```python
from build123d import *

# Parameters (mm, degrees)
BOSS_EXTRUDE1_DEPTH      = 47.064502155
BOSS_EXTRUDE1_DEPTH_BACK = 1
SKETCH1_W                = 107.713145043
SKETCH1_H                = 42.376311336
SKETCH2_R                = 13.469541987
SKETCH2_R_2              = 9.325857952
BOSS_EXTRUDE2_DEPTH      = 25.604576726
SKETCH3_OUTSIDE_W        = 137.154
SKETCH3_OUTSIDE_H        = 71.816
CUT_EXTRUDE2_DEPTH       = 12.802288363
SKETCH5_W                = 30.426797769
SKETCH5_H                = 5.633317916
CUT_EXTRUDE3_DEPTH       = 19.604576726


with BuildPart() as part:
    # Sketch1 → Boss-Extrude1 (new, two sides: drawn at the far end of the back side and taken through both)
    with BuildSketch(Plane(origin=(-41.279886751, 0, 0), x_dir=(1, 0, 0), z_dir=(0, 0, 1)).offset(-BOSS_EXTRUDE1_DEPTH_BACK)):
        with Locations((16.738942234, -3.835786802)):
            Rectangle(SKETCH1_W, SKETCH1_H)
    extrude(amount=BOSS_EXTRUDE1_DEPTH + BOSS_EXTRUDE1_DEPTH_BACK)

    # Sketch2 → Boss-Extrude2 (add)
    with BuildSketch(Plane(origin=(-44.843209588, 3.141572349, 47.064502155), x_dir=(1, 0, 0), z_dir=(0, 0, 1))):
        with Locations((1.586562206, -2.539630295)):
            Circle(SKETCH2_R)
        with Locations((1.586562206, -2.539630295)):
            Circle(SKETCH2_R_2, mode=Mode.SUBTRACT)
    extrude(amount=BOSS_EXTRUDE2_DEPTH)

    # Sketch3 outside → Cut-Extrude2 (cut, symmetric)
    with BuildSketch(Plane.XY.offset(72.669078881)):
        with Locations((-24.541, -3.836)):
            Rectangle(SKETCH3_OUTSIDE_W, SKETCH3_OUTSIDE_H)
        Polygon((-18.492947879, -30.338784684), (-15.338367542, -1.062929581), (-42.269291948, -12.968910423), align=None, mode=Mode.SUBTRACT)
    extrude(amount=CUT_EXTRUDE2_DEPTH, both=True, mode=Mode.SUBTRACT)

    # Sketch5 → Cut-Extrude3 (cut)
    with BuildSketch(Plane.XY.offset(47.064502155)):
        with Locations((7.480827718, 6.71069858)):
            Rectangle(SKETCH5_W, SKETCH5_H)
    extrude(amount=-CUT_EXTRUDE3_DEPTH, mode=Mode.SUBTRACT)


solid = part.part
```
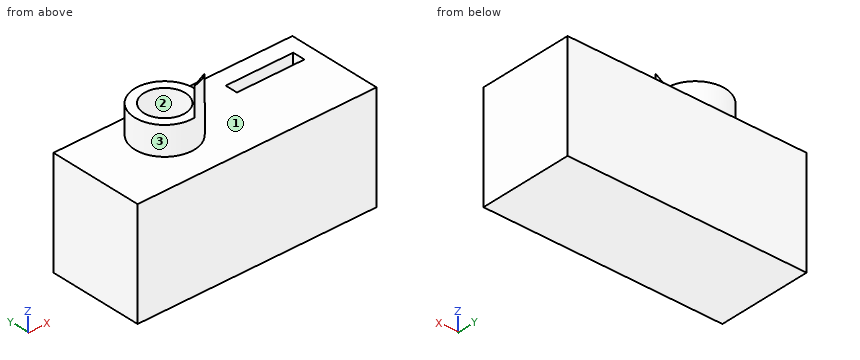
Verification items for the finished model (mm, model axes). Face numbers are marked on the shaded views. Round coordinates to 2 decimals unless told otherwise and drop trailing zeros. Write each loop counter-clockwise with the first axis right and the second up, starting at its lowest first coordinate (ties: lowest second). Pieces come first, ordered by that corner, then holes. Notation, with made-up numbers: (53, -3) - (88, -3) arc R23 ccw to (88, 35) - close; hole circle Ø7 at (80.5, 55). An arc over 180 degrees is marked (long way). Answer as a JSON object with one key per item and string values. Group by question number.
Q1. Section check A-A, the plane z = 36.5. Enter the section's corners in (x, y).
Q2. Mould release check, pull along X, two halves, no side actions. Record for the marked faces 1, 2 and 3: released by +X, released by -X, zero draft, split by the parting line, or undercut.
Q3. Section check D-D, the plane z = 68.5. Enter the section's corners in (x, y), plus the area to 3 significant figures.
Q4. Go/stop test with flat-tipped pins: pin 1 Ø8 at (x, y) = (-16, -13.5) entering from +Z; pin 2 Ø24 at (x, y) = (-43.26, 0.6) entering from +Z; pin 3 Ø6 at (y, z) = (-12.5, 53) entering from +X. Record where each tip stops, or that it passes through.
Q5. Section check B-B, the plane x = -36.5. Enter the section's corners in (y, z), plus the area to 3 significant figures.
Q6. Section check C-C, the plane y = -4. Enter the section's corners in (x, z).
Q7. Thickness scan on line 1 (Z direction, x = -8.5, y = -13); line 2 (Z direction, x = -54.5, y = 3); line 3 (X direction, y = -4, z = 59). Record the ranges inside material, lowest first.
Found:
{
 "1": {"outline": "(-78.4, -25.02) - (29.32, -25.02) - (29.32, 17.35) - (-78.4, 17.35) - close; hole (-7.73, 3.89) - (22.69, 3.89) - (22.69, 9.53) - (-7.73, 9.53) - close"},
 "2": {"face 1": "zero draft", "face 2": "undercut", "face 3": "split by the parting line"},
 "3": {"outline": "(-41.88, -12.8) arc R13.47 ccw to (-34.27, -9.43) - close", "area": "3.67 mm^2"},
 "4": {"pin 1": "stops at z = 47.06", "pin 2": "stops at z = 59.87", "pin 3": "stops at x = -34.35"},
 "5": {"outline": "(-25.02, -1) - (17.35, -1) - (17.35, 47.06) - (12.25, 47.06) - (12.25, 59.87) - (7.03, 59.87) - (7.03, 47.06) - (-5.83, 47.06) - (-5.83, 59.87) - (-10.42, 59.87) - (-10.42, 72.67) - (-11.05, 72.67) - (-11.05, 47.06) - (-25.02, 47.06) - close", "area": "2,180 mm^2"},
 "6": {"outline": "(-78.4, -1) - (29.32, -1) - (29.32, 47.06) - (-30.6, 47.06) - (-30.6, 59.87) - (-35.15, 59.87) - (-35.15, 47.06) - (-51.37, 47.06) - (-51.37, 59.87) - (-55.92, 59.87) - (-55.92, 47.06) - (-78.4, 47.06) - close"},
 "7": {"line 1": "z = -1 to 47.06", "line 2": "z = -1 to 59.87", "line 3": "x = -55.92 to -51.37, -35.15 to -30.6"}
}
